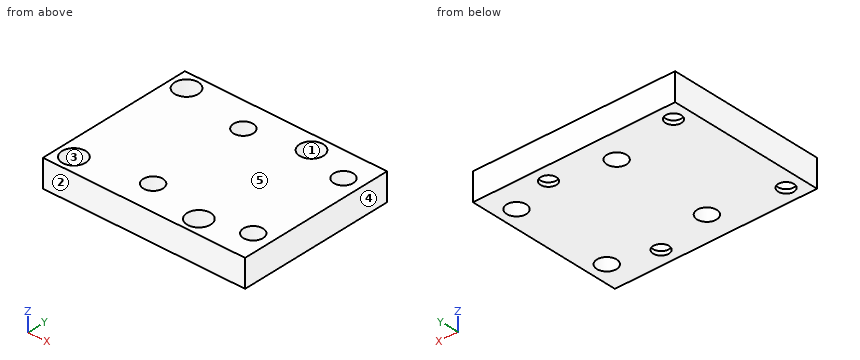
```python
from build123d import *

# Parameters (mm, degrees)
SKETCH1_W           = 51.34
SKETCH1_H           = 40
BOSS_EXTRUDE1_DEPTH = 7
SKETCH2_R           = 2
CUT_EXTRUDE2_DEPTH  = 8
SKETCH8_R           = 3
CUT_EXTRUDE6_DEPTH  = 6
SKETCH9_R           = 2.49
CUT_EXTRUDE7_DEPTH  = 7


with BuildPart() as part:
    # Sketch1 → Boss-Extrude1 (new body)
    with BuildSketch(Plane.XY):
        with Locations((-39.76, -20)):
            Rectangle(SKETCH1_W, SKETCH1_H)
    extrude(amount=BOSS_EXTRUDE1_DEPTH)

    # Sketch2 → Cut-Extrude2 (cut, through all)
    with BuildSketch(Plane.XY):
        with Locations((-61.3, -35.875)):
            Circle(SKETCH2_R)
        with Locations((-29.55, -35.875)):
            Circle(SKETCH2_R)
        with Locations((-29.55, -4.125)):
            Circle(SKETCH2_R)
        with Locations((-61.3, -4.125)):
            Circle(SKETCH2_R)
    extrude(amount=CUT_EXTRUDE2_DEPTH, mode=Mode.SUBTRACT)

    # Sketch8 → Cut-Extrude6 (cut)
    with BuildSketch(Plane.XY.offset(7)):
        with Locations((-61.3, -4.125)):
            Circle(SKETCH8_R)
        with Locations((-29.55, -4.125)):
            Circle(SKETCH8_R)
        with Locations((-29.55, -35.875)):
            Circle(SKETCH8_R)
        with Locations((-61.3, -35.875)):
            Circle(SKETCH8_R)
    extrude(amount=-CUT_EXTRUDE6_DEPTH, mode=Mode.SUBTRACT)

    # Sketch9 → Cut-Extrude7 (cut)
    with BuildSketch(Plane.XY.offset(7)):
        with Locations((-44.030806884, -7.27)):
            Circle(SKETCH9_R)
        with Locations((-18.600806884, -7.27)):
            Circle(SKETCH9_R)
        with Locations((-44.030806884, -32.7)):
            Circle(SKETCH9_R)
        with Locations((-18.600806884, -32.7)):
            Circle(SKETCH9_R)
    extrude(amount=-CUT_EXTRUDE7_DEPTH, mode=Mode.SUBTRACT)


solid = part.part
```
Part model, mm, in its own coordinate system. Face numbers are marked on the shaded views. A direction names the side the tool comes from. Round coordinates to 2 decimals unless told otherwise and drop trailing zeros. Write each loop counter-clockwise with the first axis right and the second up, starting at its lowest first coordinate (ties: lowest second). Pieces come first, ordered by that corner, then holes.
Item 1: Cut at B-B, the plane y = -9. Give the cut face in (x, z), plus the area to 3 significant figures.
Results:
outline: (-65.43, 0) - (-45.82, 0) - (-45.82, 7) - (-65.43, 7) - close; (-42.24, 0) - (-20.39, 0) - (-20.39, 7) - (-42.24, 7) - close; (-16.81, 0) - (-14.09, 0) - (-14.09, 7) - (-16.81, 7) - close
area: 309 mm2
Item 2: Which spindle directions (+Z, -Z, +X, -X, +Y, -Y) get a long thin tool onto all of the face, cutting with end or side? Do the marked faces 1 and 2. Say none if no direction does.
Results:
face 1: +Z
face 2: +Z, -Z, +X, -X, -Y
Item 3: Two-plate mould, pull along X, no slides. Class the marked faces 3, 4 and 5: +X half, -X half, draft (parallel to the pull), parting line (faces both ways), or undercut.
Results:
face 3: undercut
face 4: +X half
face 5: draft
Item 4: Drop a flat-ended pin along its axis: pin 1 Ø3 at (x, y) = (-30, -37) entering from +Z. Give the stop position or say it passes through.
Results:
pin 1: stops at z = 1
Item 5: Probe L1, parallel to Y at x = -61.3, z = 0.35 (3 decimals); L2, parallel to Y at x = -29.55, z = 5.65 (3 decimals); L3, parallel to X at y = -38, z = 6. List the from-to ranges inside material, lowest first.
Results:
L1: y = -40 to -37.875, -33.875 to -6.125, -2.125 to 0
L2: y = -40 to -38.875, -32.875 to -7.125, -1.125 to 0
L3: x = -65.43 to -63.42, -59.18 to -31.67, -27.43 to -14.09
Item 6: Cut at A-A, the plane x = -29.55. Give the cut face in (y, z) (3 decimals).
Results:
outline: (-40, 0) - (-37.875, 0) - (-37.875, 1) - (-38.875, 1) - (-38.875, 7) - (-40, 7) - close; (-33.875, 0) - (-6.125, 0) - (-6.125, 1) - (-7.125, 1) - (-7.125, 7) - (-32.875, 7) - (-32.875, 1) - (-33.875, 1) - close; (-2.125, 0) - (0, 0) - (0, 7) - (-1.125, 7) - (-1.125, 1) - (-2.125, 1) - close
Item 7: Cut at C-C, the plane z = 2. Count the separate pieces of the cut face and the enclosed holes in it, plus the area to 3 significant figures.
Results:
separate pieces: 1
enclosed holes: 8
area: 1,860 mm2
